```python
from build123d import *

# Parameters (mm, degrees)
SKETCH_1_W                = 44
SKETCH_1_H                = 34
EXTRUDE_1_DEPTH           = 24
CUT_EXTRUDE_1_DEPTH       = 31
SKETCH_5_W                = 23
SKETCH_5_H                = 6.11
EXTRUDE_4_DEPTH           = 1
EXTRUDE_5_DEPTH           = 23
SKETCH_7_R                = 1.8
CUT_EXTRUDE_2_DEPTH       = 23
CUT_EXTRUDE_4_DEPTH       = 14
SKETCH_11_R               = 1.7
EXTRUDE_6_DEPTH           = 20
CUT_EXTRUDE_7_DEPTH       = 4
CHAMFER_3_SIZE            = 2.4
SKETCH_14_W               = 40.8
SKETCH_14_H               = 4
CUT_EXTRUDE_8_DEPTH       = 23
SKETCH_15_W               = 44
SKETCH_15_H               = 1
CUT_EXTRUDE_9_DEPTH       = 24
SKETCH_16_W               = 3.2
SKETCH_16_H               = 14.6
CUT_EXTRUDE_10_DEPTH      = 5
CUT_EXTRUDE_12_DEPTH      = 10
CUT_EXTRUDE_12_DEPTH_BACK = 17
SKETCH_19_W               = 1
SKETCH_19_H               = 6.11
CUT_EXTRUDE_13_DEPTH      = 23
CHAMFER_4_SIZE            = 1.5
SKETCH_22_W               = 34
SKETCH_22_H               = 7.4
SKETCH_22_W_2             = 5.5
SKETCH_22_H_2             = 3
CUT_EXTRUDE_14_DEPTH      = 7.6
SKETCH_23_W               = 6
SKETCH_23_H               = 5.8
CUT_EXTRUDE_15_DEPTH      = 2.5
SKETCH_25_W               = 2.5
SKETCH_25_H               = 5.8
CUT_EXTRUDE_17_DEPTH      = 7
SKETCH_26_W               = 34
SKETCH_26_H               = 4
EXTRUDE_7_DEPTH           = 9
SKETCH_27_W               = 22
SKETCH_27_H               = 4.9
CUT_EXTRUDE_18_DEPTH      = 6
SKETCH_28_R               = 1.7
CUT_EXTRUDE_19_DEPTH      = 4
CHAMFER_5_SIZE            = 5
CHAMFER_5_SIZE_2          = 9.4
CHAMFER_6_SIZE            = 5
CHAMFER_6_SIZE_2          = 9.4
SKETCH_30_W               = 5
SKETCH_30_H               = 7.4
EXTRUDE_8_DEPTH           = 9.4
SKETCH_32_W               = 5
SKETCH_32_H               = 4
EXTRUDE_9_DEPTH           = 9
SKETCH_33_W               = 1.6
SKETCH_33_H               = 4
CUT_EXTRUDE_20_DEPTH      = 7.4
CHAMFER_START             = 3.158134344
CHAMFER_7_DEPTH           = 2.841865656
CHAMFER_START_2           = -6
CHAMFER_8_DEPTH           = 2.841865656
CHAMFER_START_3           = 9
CHAMFER_9_DEPTH           = 4.404008624
CHAMFER_START_4           = -13.404008624
CHAMFER_10_DEPTH          = 14.281940081
CHAMFER_11_SIZE           = 6
CHAMFER_12_SIZE           = 6


with BuildPart() as part:
    # Sketch 1 → Extrude 1 (new body)
    with BuildSketch(Plane.XY):
        with Locations((0, 27)):
            Rectangle(SKETCH_1_W, SKETCH_1_H)
    extrude(amount=EXTRUDE_1_DEPTH)

    # Sketch 2 → Cut-Extrude 1 (cut)
    with BuildSketch(Plane(origin=(0, 44, 0), x_dir=(1, 0, 0), z_dir=(0, 1, 0))):
        Polygon((-18.8, 0), (18.8, 0), (18.8, -20), (20.4, -20), (20.4, -22), (18.8, -22), (18.8, -24), (-18.8, -24), (-18.8, -22), (-20.4, -22), (-20.4, -20), (-18.8, -20), align=None)
    extrude(amount=-CUT_EXTRUDE_1_DEPTH, mode=Mode.SUBTRACT)



with BuildPart() as body_2:
    # Sketch 5 → Extrude 4 (new body)
    with BuildSketch(Plane(origin=(0, 0, 0), x_dir=(-1, 0, 0), z_dir=(0, 0, -1))):
        with Locations((0, 6.945)):
            Rectangle(SKETCH_5_W, SKETCH_5_H)
    extrude(amount=EXTRUDE_4_DEPTH)


with BuildPart() as part_1:
    add(part.part)

    add(body_2.part)  # Extrude 5 merges body 2
    # Sketch 6 → Extrude 5 (add)
    with BuildSketch(Plane(origin=(11.5, 0, 0), x_dir=(0, 0, -1), z_dir=(1, 0, 0))):
        Polygon((0, 3.89), (-7, 3.89), (-24, 10), (0, 10), align=None)
    extrude(amount=-EXTRUDE_5_DEPTH)

    # Sketch 7 → Cut-Extrude 2 (cut)
    with BuildSketch(Plane.ZY.offset(11.5)):
        with Locations(Location((3, 7.79, 0), (0, 0, 270))):
            Circle(SKETCH_7_R)
    extrude(amount=-CUT_EXTRUDE_2_DEPTH, mode=Mode.SUBTRACT)

    # Sketch 8 → Cut-Extrude 4 (cut)
    with BuildSketch(Plane.ZY.offset(7)):
        Polygon((20, 13), (-1, 13), (-1, 3.89), (10, 3.89), (10, 7.278569391), align=None)
    extrude(amount=-CUT_EXTRUDE_4_DEPTH, mode=Mode.SUBTRACT)

    # Sketch 11 → Extrude 6 (add)
    # profile 1 of 2: a face of its own
    with BuildSketch(Plane(origin=(0, 0, 0), x_dir=(-1, 0, 0), z_dir=(0, 0, -1))):
        Polygon((-14, 43), (-18.8, 43), (-18.8, 35.6), (-14, 35.6), (-10, 35.6), (-10, 43), align=None)
        with Locations((-14, 39.3)):
            Circle(SKETCH_11_R, mode=Mode.SUBTRACT)
    # profile 2 of 2: a face of its own
    with BuildSketch(Plane(origin=(0, 0, 0), x_dir=(-1, 0, 0), z_dir=(0, 0, -1))):
        Polygon((18.8, 35.6), (14, 35.6), (10, 35.6), (10, 43), (14, 43), (18.8, 43), align=None)
        with Locations((14, 39.3)):
            Circle(SKETCH_11_R, mode=Mode.SUBTRACT)
    extrude(amount=-EXTRUDE_6_DEPTH)

    # Sketch 13 → Cut-Extrude 7 (cut)
    with BuildSketch(Plane.ZY.offset(22)):
        Polygon((9, 34), (17, 36), (17, 33.5), (9, 31.5), align=None)
        Polygon((9, 30.5), (17, 32.5), (17, 30), (9, 28), align=None)
        Polygon((9, 27), (17, 29), (17, 26.5), (9, 24.5), align=None)
        Polygon((9, 23.5), (17, 25.5), (17, 23), (9, 21), align=None)
        Polygon((9, 20), (17, 22), (17, 19.5), (9, 17.5), align=None)
    cut_extrude_7 = extrude(amount=-CUT_EXTRUDE_7_DEPTH, mode=Mode.SUBTRACT)

    # Mirror 1: Cut-Extrude 7 across plane
    add(cut_extrude_7.mirror(Plane(origin=(0, 0, 0), x_dir=(0, 0, 1), z_dir=(1, 0, 0))), mode=Mode.SUBTRACT)

    # Chamfer 3
    chamfer_3_edges = [part_1.edges().sort_by_distance(p)[0] for p in [
        (22, 10, 12),
        (-22, 10, 12),
    ]]
    chamfer(chamfer_3_edges, length=CHAMFER_3_SIZE)

    # Sketch 14 → Cut-Extrude 8 (cut)
    with BuildSketch(Plane(origin=(0, 44, 0), x_dir=(1, 0, 0), z_dir=(0, 1, 0))):
        with Locations((0, -22)):
            Rectangle(SKETCH_14_W, SKETCH_14_H)
    extrude(amount=-CUT_EXTRUDE_8_DEPTH, mode=Mode.SUBTRACT)

    # Sketch 15 → Cut-Extrude 9 (cut)
    with BuildSketch(Plane(origin=(0, 0, 0), x_dir=(-1, 0, 0), z_dir=(0, 0, -1))):
        with Locations((0, 43.5)):
            Rectangle(SKETCH_15_W, SKETCH_15_H)
    extrude(amount=-CUT_EXTRUDE_9_DEPTH, mode=Mode.SUBTRACT)

    # Sketch 16 → Cut-Extrude 10 (cut)
    with BuildSketch(Plane.XY.offset(24)):
        with Locations((20.4, 28.3)):
            Rectangle(SKETCH_16_W, SKETCH_16_H)
    extrude(amount=-CUT_EXTRUDE_10_DEPTH, mode=Mode.SUBTRACT)

    # Sketch 18 → Cut-Extrude 12 (cut, two sides: drawn at the far end of the back side and taken through both)
    with BuildSketch(Plane(origin=(0, 0, 0), x_dir=(-1, 0, 0), z_dir=(0, 0, -1)).offset(-CUT_EXTRUDE_12_DEPTH_BACK)):
        Polygon((-22, 43), (-17, 43), (-17, 10), (-19.6, 10), (-22, 12.4), align=None)
        Polygon((22, 12.4), (19.6, 10), (17, 10), (17, 43), (22, 43), align=None)
    extrude(amount=CUT_EXTRUDE_12_DEPTH + CUT_EXTRUDE_12_DEPTH_BACK, mode=Mode.SUBTRACT)

    # Sketch 19 → Cut-Extrude 13 (cut)
    with BuildSketch(Plane.ZY.offset(11.5)):
        with Locations((-0.5, 6.945)):
            Rectangle(SKETCH_19_W, SKETCH_19_H)
    extrude(amount=-CUT_EXTRUDE_13_DEPTH, mode=Mode.SUBTRACT)

    # Chamfer 4
    chamfer_4_edges = [part_1.edges().sort_by_distance(p)[0] for p in [
        (-9.25, 3.89, 0),
        (9.25, 3.89, 0),
    ]]
    chamfer(chamfer_4_edges, length=CHAMFER_4_SIZE)

    # Sketch 22 → Cut-Extrude 14 (cut)
    with BuildSketch(Plane(origin=(0, 0, 0), x_dir=(-1, 0, 0), z_dir=(0, 0, -1))):
        with Locations((0, 39.3)):
            Rectangle(SKETCH_22_W, SKETCH_22_H)
        with Locations((-14.25, 11.5)):
            Rectangle(SKETCH_22_W_2, SKETCH_22_H_2)
        with Locations((14.25, 11.5)):
            Rectangle(SKETCH_22_W_2, SKETCH_22_H_2)
    extrude(amount=-CUT_EXTRUDE_14_DEPTH, mode=Mode.SUBTRACT)

    # Sketch 23 → Cut-Extrude 15 (cut)
    with BuildSketch(Plane(origin=(-7, 0, 0), x_dir=(0, 0, -1), z_dir=(1, 0, 0))):
        with Locations((-3, 7.79)):
            Rectangle(SKETCH_23_W, SKETCH_23_H)
        Polygon((-20, 13), (-10, 7.278569391), (-10, 13), align=None)
    cut_extrude_15 = extrude(amount=-CUT_EXTRUDE_15_DEPTH, mode=Mode.SUBTRACT)

    # Mirror 2: Cut-Extrude 15 across plane
    add(cut_extrude_15.mirror(Plane(origin=(0, 0, 0), x_dir=(0, 0, 1), z_dir=(1, 0, 0))), mode=Mode.SUBTRACT)

    # Sketch 25 → Cut-Extrude 17 (cut)
    with BuildSketch(Plane(origin=(17, 0, 0), x_dir=(0, 0, -1), z_dir=(1, 0, 0))):
        with Locations((-11.25, 39.3)):
            Rectangle(SKETCH_25_W, SKETCH_25_H)
    cut_extrude_17 = extrude(amount=-CUT_EXTRUDE_17_DEPTH, mode=Mode.SUBTRACT)

    # Mirror 3: Cut-Extrude 17 across plane
    add(cut_extrude_17.mirror(Plane(origin=(0, 0, 0), x_dir=(0, 0, 1), z_dir=(1, 0, 0))), mode=Mode.SUBTRACT)

    # Sketch 26 → Extrude 7 (add)
    with BuildSketch(Plane(origin=(0, 43, 0), x_dir=(1, 0, 0), z_dir=(0, 1, 0))):
        with Locations((0, -9.6)):
            Rectangle(SKETCH_26_W, SKETCH_26_H)
    extrude(amount=EXTRUDE_7_DEPTH)

    # Sketch 27 → Cut-Extrude 18 (cut)
    with BuildSketch(Plane(origin=(0, 52, 0), x_dir=(1, 0, 0), z_dir=(0, 1, 0))):
        with Locations((0, -10.05)):
            Rectangle(SKETCH_27_W, SKETCH_27_H)
    extrude(amount=-CUT_EXTRUDE_18_DEPTH, mode=Mode.SUBTRACT)

    # Sketch 28 → Cut-Extrude 19 (cut)
    with BuildSketch(Plane.XY.offset(11.6)):
        with Locations((-14, 48.3)):
            Circle(SKETCH_28_R)
        with Locations(Location((14, 48.3, 0), (0, 0, 180))):
            Circle(SKETCH_28_R)
    extrude(amount=-CUT_EXTRUDE_19_DEPTH, mode=Mode.SUBTRACT)

    # Chamfer 5
    # the kernel refuses this chamfer: 9.4, 5 mm, written as the material it adds along each edge
    with BuildSketch(Plane(origin=(-17, 10, 17), x_dir=(-1, 0, 0), z_dir=(0, 1, 0))) as chamfer_5_piece_1_section:
        Polygon((CHAMFER_5_SIZE, 0), (0, -CHAMFER_5_SIZE_2), (0, 0), align=None)
    chamfer_5_piece_1 = extrude(amount=3, mode=Mode.PRIVATE)
    chamfer_5_piece_1 = split(chamfer_5_piece_1, bisect_by=Plane(origin=(-18.3, 8.7, 17), z_dir=(0.7071067811865478, 0.7071067811865474, 0)), keep=Keep.TOP, mode=Mode.PRIVATE)
    add(chamfer_5_piece_1)

    # Chamfer 6
    # the kernel refuses this chamfer: 9.4, 5 mm, written as the material it adds along each edge
    with BuildSketch(Plane(origin=(17, 13, 17), x_dir=(1, 0, 0), z_dir=(0, -1, 0))) as chamfer_6_piece_1_section:
        Polygon((CHAMFER_6_SIZE, 0), (0, -CHAMFER_6_SIZE_2), (0, 0), align=None)
    chamfer_6_piece_1 = extrude(amount=3, mode=Mode.PRIVATE)
    chamfer_6_piece_1 = split(chamfer_6_piece_1, bisect_by=Plane(origin=(19.8, 10.2, 17), z_dir=(-0.7071067811865478, 0.7071067811865474, 0)), keep=Keep.TOP, mode=Mode.PRIVATE)
    add(chamfer_6_piece_1)

    # Sketch 30 → Extrude 8 (add)
    with BuildSketch(Plane(origin=(0, 0, 7.6), x_dir=(-1, 0, 0), z_dir=(0, 0, -1))):
        with Locations((-19.5, 39.3)):
            Rectangle(SKETCH_30_W, SKETCH_30_H)
        with Locations((19.5, 39.3)):
            Rectangle(SKETCH_30_W, SKETCH_30_H)
    extrude(amount=-EXTRUDE_8_DEPTH)

    # Sketch 32 → Extrude 9 (add)
    with BuildSketch(Plane(origin=(0, 52, 0), x_dir=(1, 0, 0), z_dir=(0, 1, 0))):
        with Locations((-19.5, -9.6)):
            Rectangle(SKETCH_32_W, SKETCH_32_H)
        with Locations((19.5, -9.6)):
            Rectangle(SKETCH_32_W, SKETCH_32_H)
    extrude(amount=-EXTRUDE_9_DEPTH)

    # Sketch 33 → Cut-Extrude 20 (cut)
    with BuildSketch(Plane(origin=(0, 43, 0), x_dir=(1, 0, 0), z_dir=(0, 1, 0))):
        with Locations((21.2, -22)):
            Rectangle(SKETCH_33_W, SKETCH_33_H)
    extrude(amount=-CUT_EXTRUDE_20_DEPTH, mode=Mode.SUBTRACT)

    # Chamfer 7: read off the stored shape, not the designer's step
    # Chamfer 7 outline → Chamfer 7 (cut)
    with BuildSketch(Plane(origin=(0, 0, 0), x_dir=(0.6735542111960274, -0.35393772244377236, -0.648885824480249), z_dir=(0.7391378251585405, 0.3225328691600908, 0.5913102601268327)).offset(CHAMFER_START)):
        Polygon((-13.858270642, 1.79569549), (-13.858270642, 8.060677533), (-17.421458222, 6.624121141), align=None)
    extrude(amount=CHAMFER_7_DEPTH, mode=Mode.SUBTRACT)

    # Chamfer 8: read off the stored shape, not the designer's step
    # Chamfer 8 outline → Chamfer 8 (cut)
    with BuildSketch(Plane(origin=(0, 0, 0), x_dir=(0.6735542111960274, 0.35393772244377236, 0.648885824480249), z_dir=(0.7391378251585405, -0.3225328691600908, -0.5913102601268327)).offset(CHAMFER_START_2)):
        Polygon((17.421458222, -6.624121141), (13.858270642, -1.79569549), (13.858270642, -8.060677533), align=None)
    extrude(amount=CHAMFER_8_DEPTH, mode=Mode.SUBTRACT)

    # Chamfer 9: read off the stored shape, not the designer's step
    # Chamfer 9 outline → Chamfer 9 (cut)
    with BuildSketch(Plane(origin=(0, 0, 0), x_dir=(0.7291332431365165, -0.583961995177201, -0.35686566371940037), z_dir=(0.6843717657481387, 0.6221561506801269, 0.3802065365267439)).offset(CHAMFER_START_3)):
        Polygon((-42.753948395, 4.399141898), (-35.896491206, 12.078678401), (-42.753948395, 14.946653453), align=None)
    extrude(amount=CHAMFER_9_DEPTH, mode=Mode.SUBTRACT)

    # Chamfer 10: read off the stored shape, not the designer's step
    # Chamfer 10 outline → Chamfer 10 (cut)
    with BuildSketch(Plane(origin=(0, 0, 0), x_dir=(0.7291332431365165, 0.583961995177201, 0.35686566371940037), z_dir=(0.6843717657481387, -0.6221561506801269, -0.3802065365267439)).offset(CHAMFER_START_4)):
        Polygon((42.753948395, -4.399141898), (35.896491206, -12.078678401), (42.753948395, -14.946653453), align=None)
    extrude(amount=CHAMFER_10_DEPTH, mode=Mode.SUBTRACT)

    # Chamfer 11
    chamfer_11_edges = [part_1.edges().sort_by_distance(p)[0] for p in [
        (-20.4, 13, 17),
    ]]
    chamfer(chamfer_11_edges, length=CHAMFER_11_SIZE)

    # Chamfer 12
    chamfer_12_edges = [part_1.edges().sort_by_distance(p)[0] for p in [
        (20.4, 13, 17),
    ]]
    chamfer(chamfer_12_edges, length=CHAMFER_12_SIZE)


solid = part_1.part
```
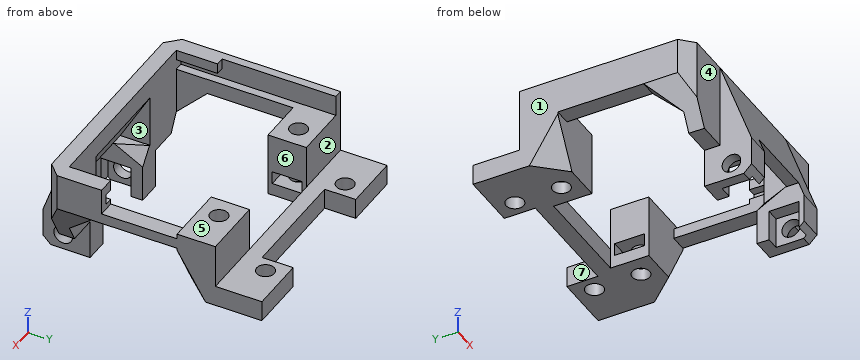
Part model, mm, in its own coordinate system. Face numbers are marked on the shaded views. A direction names the side the tool comes from. Give positions to 0.01 mm unless a question says otherwise; leave off trailing zeros. Order: outer loops, then holes, each group sorted by start corner. A loop starts at its lowest first (then second) coordinate and runs counter-clockwise, first axis right, second up. Notation, with made-up numbers: M 89.5,-14 L 144.5,-14 A24 cw 144.5,8 Z; hole C 46,39.5 d4. An arc over 180 degrees is marked long. Use a Markdown table: item, result. Add a question column.
(1) Saw through at A-A, the plane z = 3. Give the cut face in (x, y).
(2) Drop flat-ended pins along their axis: P1, Ø5, axis at x = -11, y = 44, coming from the +Z side; P2, Ø4.5, axis at x = -14, y = 39.3, coming from the -Z side; P3, Ø1.5, axis at x = 4.5, y = 47, coming from the -Z side; P4, Ø1.2, axis at x = -15, z = 11.5, coming from the -Y side. Give the stop position or say it passes through.
(3) Saw through at C-C, the plane x = -14. Give the cut face in (y, z).
(4) Probe line 1 along Y through (x, z) = (-14, 18.5); line 2 along Y through (x, z) = (11, 12); line 3 along X through (y, z) = (34, 21.75). List the from-to ranges inside material, lowest first. Write a range as [from, to].
(5) Mould opens along X. For the marked faces 1, 2 and 3 say: +X half, -X half, draft (parallel to the pull), parting line (faces both ways), or undercut.
(6) Saw through at B-B, the plane x = -6. Give the cut face in (y, z), and give its area (3 significant figures).
(7) Saw through at D-D, the plane z = 9. Give the number of separate pieces and of enclosed holes in the cut face, and give its area (3 significant figures).
(8) 3-axis set-ups, long thin cutter, end or side, ignore diameter. For the marked faces 4, 5, 6 and 7: which of +Z, -Z, +X, -X, +Y, -Y reach the whole face in a straight line?
Answer key:
| question | item | result |
|---|---|---|
| 1 | outline | M -11.5,3.89 L -7,3.89 L -7,4.89 L -9.5,4.89 L -9.5,5.99 L -11.5,5.99 Z; M -11.5,9.59 L -9.5,9.59 L -9.5,10.69 L -7,10.69 L -7,13 L -11.5,13 Z; M 7,3.89 L 11.5,3.89 L 11.5,5.99 L 9.5,5.99 L 9.5,4.89 L 7,4.89 Z; M 7,10.69 L 9.5,10.69 L 9.5,9.59 L 11.5,9.59 L 11.5,13 L 7,13 Z |
| 2 | P1 | z = 20 |
| 2 | P2 | z = 7.6 |
| 2 | P3 | through |
| 2 | P4 | y = 10 |
| 3 | outline | M 10,7.6 L 13,7.6 L 13,24 L 10,24 Z; M 35.6,7.6 L 37.6,7.6 L 37.6,10 L 36.4,10 L 36.4,12.5 L 37.6,12.5 L 37.6,20 L 35.6,20 Z; M 41,7.6 L 46.6,7.6 L 46.6,11.6 L 43,11.6 L 43,20 L 41,20 L 41,12.5 L 42.2,12.5 L 42.2,10 L 41,10 Z; M 50,7.6 L 52,7.6 L 52,11.6 L 50,11.6 Z |
| 4 | line 1 | [10, 13], [35.6, 37.6], [41, 43] |
| 4 | line 2 | [5.69, 13], [35.6, 36.4], [42.2, 43] |
| 4 | line 3 | [-22, -20.4] |
| 5 | face 1 | -X half |
| 5 | face 2 | draft |
| 5 | face 3 | undercut |
| 6 | outline | M 4.97,10 L 7.28,10 L 13,20 L 13,24 L 10,24 Z; M 43,7.6 L 46,7.6 L 46,11.6 L 43,11.6 Z |
| 6 | area | 60.6 mm^2 |
| 7 | separate pieces | 3 |
| 7 | enclosed holes | 4 |
| 7 | area | 493 mm^2 |
| 8 | face 4 | +Z, -Z, -X, -Y |
| 8 | face 5 | +Z, +X, +Y |
| 8 | face 6 | +Z, -Z |
| 8 | face 7 | +Z, -Z, +Y |
